```python
from build123d import *

# Parameters (mm, degrees)
F1_DEPTH  = 125
F2_R      = 1.85
F3_DEPTH  = 4
F5_DEPTH  = 3
F7_R      = 6
F8_DEPTH  = 25
F10_R     = 6
F11_DEPTH = 25


with BuildPart() as f1:
    # F0 (on Front) → F1 (new body)
    with BuildSketch(Plane.XZ):
        Polygon((27.4241377865, 47.5), (-27.4241377865, 47.5), (-23.9600361714, 41.5), (23.9600361714, 41.5), align=None)
    extrude(amount=F1_DEPTH)

    # F2 (on face) → F3 (cut)
    with BuildSketch(Plane(origin=(0, 0, 41.5), x_dir=(1, 0, 0), z_dir=(0, 0, -1))):
        with BuildLine():
            ThreePointArc((-13.8300180857, 120), (-11.9800180857, 118.15), (-10.1300180857, 120))
            Line((-10.1300180857, 120), (-13.8300180857, 120))
        make_face()
        with BuildLine():
            Line((-13.8300180857, 120), (-10.1300180857, 120))
            ThreePointArc((-10.1300180857, 120), (-11.9800180857, 121.85), (-13.8300180857, 120))
        make_face()
        with Locations((11.9800180857, 120)):
            Circle(F2_R)
        with BuildLine():
            ThreePointArc((-13.8300180857, 23), (-11.9800180857, 21.15), (-10.1300180857, 23))
            Line((-10.1300180857, 23), (-13.8300180857, 23))
        make_face()
        with BuildLine():
            Line((-13.8300180857, 23), (-10.1300180857, 23))
            ThreePointArc((-10.1300180857, 23), (-11.9800180857, 24.85), (-13.8300180857, 23))
        make_face()
        with Locations((11.9800180857, 23)):
            Circle(F2_R)
    extrude(amount=-F3_DEPTH, mode=Mode.SUBTRACT)

    # F4 (on face) → F5 (join)
    with BuildSketch(Plane.XY.offset(47.5)):
        with BuildLine():
            ThreePointArc((-4.9624431031, -72.4009279721), (4.252691201, -72.2658826822), (8.8217126606, -64.2620723161))
            Line((8.8217126606, -64.2620723161), (3.1603222234, -64.2620723161))
            ThreePointArc((3.1603222234, -64.2620723161), (0.7821935357, -70.0114263654), (-4.9624431031, -72.4009279721))
        make_face()
        with BuildLine():
            ThreePointArc((6.5204872228, -58.1396910508), (6.4966065006, -58.1411162683), (6.4727028262, -58.142082959))
            ThreePointArc((6.4727028262, -58.142082959), (6.1878056278, -58.118065532), (5.9158733115, -58.0297701993))
            ThreePointArc((5.9158733115, -58.0297701993), (5.1682662368, -59.4962219445), (3.5931775857, -59.0182127392))
            ThreePointArc((3.5931775857, -59.0182127392), (2.8253831829, -59.5446151282), (1.9358127946, -59.8189730046))
            ThreePointArc((1.9358127946, -59.8189730046), (1.892061339, -59.8251878066), (1.8482256331, -59.8307774863))
            ThreePointArc((1.8482256331, -59.8307774863), (2.8254071893, -61.9513380534), (3.1603222234, -64.2620723161))
            Line((3.1603222234, -64.2620723161), (8.8217126606, -64.2620723161))
            ThreePointArc((8.8217126606, -64.2620723161), (8.227406593, -60.991782158), (6.5204872228, -58.1396910508))
        make_face()
        with BuildLine():
            ThreePointArc((-4.9624431031, -56.1232166602), (1.0988983628, -55.1011074623), (6.4727028262, -58.0855325605))
            ThreePointArc((6.4727028262, -58.0855325605), (6.4966476292, -58.1125653923), (6.5204872228, -58.1396910508))
            ThreePointArc((6.5204872228, -58.1396910508), (7.5840164309, -57.3778876345), (7.3813630468, -56.0854595214))
            ThreePointArc((7.3813630468, -56.0854595214), (8.5743392283, -55.7885482621), (9.416500561, -54.8929407838))
            Line((9.416500561, -54.8929407838), (9.416500561, -54.2620723161))
            Line((9.416500561, -54.2620723161), (-7.6202011075, -54.2620723161))
            ThreePointArc((-7.6202011075, -54.2620723161), (-7.6869328379, -54.3259904491), (-7.7511294791, -54.3924542951))
            ThreePointArc((-7.7511294791, -54.3924542951), (-9.4471027568, -54.7050419938), (-10.1823136256, -56.265010393))
            ThreePointArc((-10.1823136256, -56.265010393), (-10.2763805171, -56.3286177025), (-10.3628188483, -56.4022579415))
            Line((-10.3628188483, -56.4022579415), (-10.3628188483, -57.883753756))
            ThreePointArc((-10.3628188483, -57.883753756), (-9.9403916974, -58.1260840744), (-9.453785384, -58.1456538666))
            ThreePointArc((-9.453785384, -58.1456538666), (-9.0506628028, -58.7755881179), (-8.3467504152, -59.0282387207))
            ThreePointArc((-8.3467504152, -59.0282387207), (-6.1696577071, -59.4019534475), (-4.3527629056, -58.1456538666))
            ThreePointArc((-4.3527629056, -58.1456538666), (-2.6797742551, -59.371466197), (-0.6360720047, -59.0182127392))
            ThreePointArc((-0.6360720047, -59.0182127392), (0.5161185349, -59.6995293687), (1.8482256331, -59.8307774863))
            ThreePointArc((1.8482256331, -59.8307774863), (1.8330187957, -59.8074376583), (1.817732163, -59.7841500149))
            ThreePointArc((1.817732163, -59.7841500149), (-1.111668826, -57.1004757298), (-4.9624431031, -56.1232166602))
        make_face()
        with BuildLine():
            Line((9.416500561, -54.2620723161), (9.416500561, -54.8929407838))
            ThreePointArc((9.416500561, -54.8929407838), (9.352384363, -52.8082417308), (7.5650540132, -51.7332853367))
            ThreePointArc((7.5650540132, -51.7332853367), (5.1359618237, -51.2192554799), (3.4312824519, -53.0244656611))
            ThreePointArc((3.4312824519, -53.0244656611), (0.771209683, -52.2310388329), (-1.2286664372, -54.1561385113))
            ThreePointArc((-1.2286664372, -54.1561385113), (-2.8757088862, -53.5841315132), (-4.5227513352, -54.1561385113))
            ThreePointArc((-4.5227513352, -54.1561385113), (-6.0911184928, -53.634775536), (-7.6202011075, -54.2620723161))
            Line((-7.6202011075, -54.2620723161), (9.416500561, -54.2620723161))
        make_face()
        with BuildLine():
            Line((1.9358127946, -59.8189730046), (1.817732163, -59.7841500149))
            ThreePointArc((1.817732163, -59.7841500149), (1.8330187957, -59.8074376583), (1.8482256331, -59.8307774863))
            ThreePointArc((1.8482256331, -59.8307774863), (1.892061339, -59.8251878066), (1.9358127946, -59.8189730046))
        make_face()
        with BuildLine():
            Line((6.4727028262, -58.0855325605), (6.4727028262, -58.142082959))
            ThreePointArc((6.4727028262, -58.142082959), (6.4966065006, -58.1411162683), (6.5204872228, -58.1396910508))
            ThreePointArc((6.5204872228, -58.1396910508), (6.4966476292, -58.1125653923), (6.4727028262, -58.0855325605))
        make_face()
    extrude(amount=F5_DEPTH)

    # F7 (on face) → F8 (cut)
    with BuildSketch(Plane(origin=(-23.9600361714, 0, 41.5), x_dir=(0.8660254038, 0, 0.5), z_dir=(0.5, 0, -0.8660254038))):
        with Locations((0, 62.5)):
            Circle(F7_R)
    extrude(amount=F8_DEPTH, mode=Mode.SUBTRACT)

    # F10 (on face) → F11 (cut)
    with BuildSketch(Plane(origin=(23.9600361714, 0, 41.5), x_dir=(0.8660254038, 0, -0.5), z_dir=(0.5, 0, 0.8660254038))):
        with Locations((0, -62.5)):
            Circle(F10_R)
    extrude(amount=-F11_DEPTH, mode=Mode.SUBTRACT)


solid = f1.part
```
The listing builds one solid part. Answer for the finished solid, in the listing's coordinates (mm). A direction names the side the tool comes from. Round coordinates to 2 decimals unless told otherwise and drop trailing zeros. Loops run counter-clockwise (first coordinate to the right, second up) from the corner with the lowest first, then second, coordinate; pieces in that order, holes last.
Q1. Find the intervals of material crossed by line 1 (X direction, y = -120, z = 43.35); line 2 (X direction, y = -23, z = 45); line 3 (Z direction, x = -2.5, y = -11), in increasing order.
Q2. Section B-B, the plane y = -23 is taken. Determine the outline of the cut face in (x, z).
Q3. Section C-C, the plane x = 0.5 is taken. Determine the outline of the cut face in (y, z), then the cut area to 3 significant figures.
Q4. For a pull along Y with two mould halves and no side action, classify faces 1 (the face through (0, -125, 45)), 2 (the face through (-25.716, -61.625, 44.542)), 3 (the face through (0, 0, 45)), 4 (the face through (11.739, -24.834, 43.472)) as released by +Y, released by -Y, zero draft, split by the parting line, or undercut.
Q5. Given pin 1 Ø3 at (x, y) = (-11.98, -23) entering from -Z; pin 2 Ø4 at (x, y) = (11, -119) entering from -Z; pin 3 Ø1.5 at (x, y) = (10, -30.5) entering from +Z, each flat-ended and moving along its own axis, determine where each tip first touches the part or whether it passes through.
Q6. Section A-A, the plane z = 48.75 is taken. Determine the outline of the cut face in (x, y).
Q7. Section D-D, the plane z = 42.75 is taken. Count the separate pieces of the cut face and the enclosed holes in it, then the cut area to 3 significant figures.
Q8. Which of the six approach directions +Z, -Z, +X, -X, +Y, -Y give full straight-line access (tool end or side, diameter ignored) to faces 5 (the face through (0, -62, 41.5)), 6 (the face through (21.9, -62.42, 42.69)), 7 (the face through (0.498, -59.694, 48.979))?
Completed:
1. line 1: x = -25.03 to -13.83, -10.13 to 10.13, 13.83 to 25.03
1. line 2: x = -25.98 to -13.83, -10.13 to 10.13, 13.83 to 25.98
1. line 3: z = 41.5 to 47.5
2. outline: (-27.42, 47.5) - (-23.96, 41.5) - (-13.83, 41.5) - (-13.83, 45.5) - (-10.13, 45.5) - (-10.13, 41.5) - (10.13, 41.5) - (10.13, 45.5) - (13.83, 45.5) - (13.83, 41.5) - (23.96, 41.5) - (27.42, 47.5) - close
3. outline: (-125, 41.5) - (0, 41.5) - (0, 47.5) - (-52.31, 47.5) - (-52.31, 50.5) - (-55.02, 50.5) - (-55.02, 47.5) - (-58.24, 47.5) - (-58.24, 50.5) - (-59.69, 50.5) - (-59.69, 47.5) - (-70.28, 47.5) - (-70.28, 50.5) - (-73.51, 50.5) - (-73.51, 47.5) - (-125, 47.5) - close
3. area: 772 mm2
4. face 1: released by -Y
4. face 2: zero draft
4. face 3: released by +Y
4. face 4: undercut
5. pin 1: stops at z = 45.5
5. pin 2: stops at z = 41.5
5. pin 3: stops at z = 47.5
6. outline: (-10.36, -57.88) arc R1.02 ccw to (-9.45, -58.15) arc R1.16 ccw to (-8.35, -59.03) arc R2.92 ccw to (-4.35, -58.15) arc R2.65 ccw to (-0.64, -59.02) arc R3.1 ccw to (1.85, -59.83) arc R8.14 cw to (-4.96, -72.4) arc R9.29 ccw to (6.52, -58.14) arc R1.25 ccw to (7.38, -56.09) arc R2.18 ccw to (7.57, -51.73) arc R2.54 ccw to (3.43, -53.02) arc R2.75 ccw to (-1.23, -54.16) arc R2.66 ccw to (-4.52, -54.16) arc R2.38 ccw to (-7.75, -54.39) arc R1.89 ccw to (-10.18, -56.27) arc R1.02 ccw to (-10.36, -56.4) - close; hole (-4.96, -56.12) arc R8.14 cw to (1.82, -59.78) - (1.94, -59.82) arc R3.1 ccw to (3.59, -59.02) arc R1.28 ccw to (5.92, -58.03) arc R1.25 ccw to (6.47, -58.14) - (6.47, -58.09) arc R9.29 ccw to start
7. separate pieces: 1
7. enclosed holes: 6
7. area: 6,060 mm2
8. face 5: -Z, +X, -X, +Y, -Y
8. face 6: -Z
8. face 7: +Z
